The listing builds one solid part. Answer for the finished solid, in the listing's coordinates (mm). Face numbers are marked on the shaded views. Round coordinates to 2 decimals unless told otherwise and drop trailing zeros. Write each loop counter-clockwise with the first axis right and the second up, starting at its lowest first coordinate (ties: lowest second). Pieces come first, ordered by that corner, then holes.
from build123d import *

# Parameters (mm, degrees)
SKETCH1_R                = 36
BOSS_EXTRUDE1_DEPTH      = 5
SKETCH2_R                = 15
CUT_EXTRUDE1_DEPTH       = 5
CUT_EXTRUDE3_DEPTH       = 5
FILLET1_R                = 1.5
CIRPATTERN1_COUNT        = 6
FILLET1_OF_CIRPATTERN1_R = 1.5
SKETCH4_R                = 1.55
CUT_EXTRUDE4_DEPTH       = 5
CIRPATTERN2_COUNT        = 8
BOSS_EXTRUDE2_DEPTH      = 2
CIRPATTERN3_COUNT        = 4


with BuildPart() as part:
    # Sketch1 → Boss-Extrude1 (new body)
    with BuildSketch(Plane(origin=(0, 0, 0), x_dir=(1, 0, 0), z_dir=(0, 1, 0))):
        with Locations(Location((0, 0, 0), (0, 0, 270))):
            Circle(SKETCH1_R)
    extrude(amount=BOSS_EXTRUDE1_DEPTH)

    # Sketch2 → Cut-Extrude1 (cut)
    with BuildSketch(Plane(origin=(0, 5, 0), x_dir=(1, 0, 0), z_dir=(0, 1, 0))):
        with Locations(Location((0, 0, 0), (0, 0, 270))):
            Circle(SKETCH2_R)
    extrude(amount=-CUT_EXTRUDE1_DEPTH, mode=Mode.SUBTRACT)

    # Sketch3 → Cut-Extrude3 (cut)
    with BuildSketch(Plane(origin=(0, 5, 0), x_dir=(1, 0, 0), z_dir=(0, 1, 0))):
        with BuildLine():
            Line((-15.909902577, 15.909902577), (-19.445436483, 19.445436483))
            ThreePointArc((-19.445436483, 19.445436483), (-13.75, 23.815698604), (-7.11752374, 26.562960223))
            Line((-7.11752374, 26.562960223), (-5.823428515, 21.733331092))
            ThreePointArc((-5.823428515, 21.733331092), (-11.25, 19.485571585), (-15.909902577, 15.909902577))
        make_face()
    cut_extrude3 = extrude(amount=-CUT_EXTRUDE3_DEPTH, mode=Mode.SUBTRACT)

    # Fillet1
    fillet1_edges = [part.edges().sort_by_distance(p)[0] for p in [
        (-19.445436483, 2.5, -19.445436483),
        (-7.11752374, 2.5, -26.562960223),
        (-5.823428515, 2.5, -21.733331092),
        (-15.909902577, 2.5, -15.909902577),
    ]]
    fillet(fillet1_edges, radius=FILLET1_R)

    # CirPattern1: Cut-Extrude3 ×6 about axis
    cirpattern1_axis = Axis((0, 0, 0), (0, 1, 0))
    for i in range(1, CIRPATTERN1_COUNT):
        add(cut_extrude3.rotate(cirpattern1_axis, i * 360 / CIRPATTERN1_COUNT), mode=Mode.SUBTRACT)

    # Fillet1 of CirPattern1
    fillet1_of_cirpattern1_edges = [part.edges().sort_by_distance(p)[0] for p in [
        (-26.562960223, 2.5, 7.11752374),
        (-26.562960223, 2.5, -7.11752374),
        (-21.733331092, 2.5, -5.823428515),
        (-21.733331092, 2.5, 5.823428515),
        (-7.11752374, 2.5, 26.562960223),
        (-19.445436483, 2.5, 19.445436483),
        (-15.909902577, 2.5, 15.909902577),
        (-5.823428515, 2.5, 21.733331092),
        (19.445436483, 2.5, 19.445436483),
        (7.11752374, 2.5, 26.562960223),
        (5.823428515, 2.5, 21.733331092),
        (15.909902577, 2.5, 15.909902577),
        (26.562960223, 2.5, -7.11752374),
        (26.562960223, 2.5, 7.11752374),
        (21.733331092, 2.5, 5.823428515),
        (21.733331092, 2.5, -5.823428515),
        (7.11752374, 2.5, -26.562960223),
        (19.445436483, 2.5, -19.445436483),
        (15.909902577, 2.5, -15.909902577),
        (5.823428515, 2.5, -21.733331092),
    ]]
    fillet(fillet1_of_cirpattern1_edges, radius=FILLET1_OF_CIRPATTERN1_R)

    # Sketch4 → Cut-Extrude4 (cut)
    with BuildSketch(Plane(origin=(0, 5, 0), x_dir=(1, 0, 0), z_dir=(0, 1, 0))):
        with Locations(Location((0, 33, 0), (0, 0, 270))):
            Circle(SKETCH4_R)
    cut_extrude4 = extrude(amount=-CUT_EXTRUDE4_DEPTH, mode=Mode.SUBTRACT)

    # CirPattern2: Cut-Extrude4 ×8 about axis
    cirpattern2_axis = Axis((0, 0, 0), (0, 1, 0))
    for i in range(1, CIRPATTERN2_COUNT):
        add(cut_extrude4.rotate(cirpattern2_axis, i * 360 / CIRPATTERN2_COUNT), mode=Mode.SUBTRACT)

    # Sketch6 → Boss-Extrude2 (add)
    with BuildSketch(Plane(origin=(0, 5, 0), x_dir=(1, 0, 0), z_dir=(0, 1, 0))):
        with BuildLine():
            Line((-16.387638055, 25.723439097), (-17.40850731, 27.325882844))
            ThreePointArc((-17.40850731, 27.325882844), (-12.398943209, 29.933696853), (-7.012643492, 31.631990631))
            Line((-7.012643492, 31.631990631), (-6.601408225, 29.777028217))
            ThreePointArc((-6.601408225, 29.777028217), (-11.671844687, 28.178325742), (-16.387638055, 25.723439097))
        make_face()
    boss_extrude2 = extrude(amount=BOSS_EXTRUDE2_DEPTH)

    # CirPattern3: Boss-Extrude2 ×4 about axis
    cirpattern3_axis = Axis((0, 5, 0), (0, -1, 0))
    for i in range(1, CIRPATTERN3_COUNT):
        add(boss_extrude2.rotate(cirpattern3_axis, i * 360 / CIRPATTERN3_COUNT))


solid = part.part
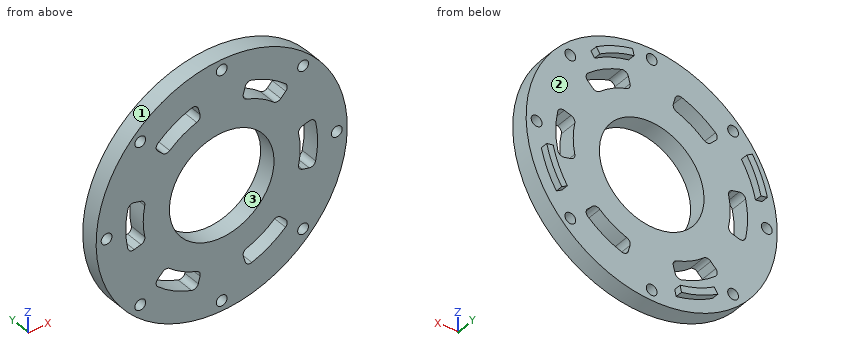
1. For a pull along Z with two mould halves and no side action, classify the marked faces 1, 2 and 3 as released by +Z, released by -Z, zero draft, split by the parting line, or undercut.
Geometry says:
face 1: split by the parting line
face 2: zero draft
face 3: undercut
2. Given pin 1 (1.5 mm diameter, centred on y = 6, z = 13.5, fed in from +X); pin 2 (4 mm diameter, centred on x = 23.33, z = 23.33, fed in from +Y); pin 3 (4 mm diameter, centred on y = 1.5, z = 27, fed in from -X), each flat-ended and moving along its own axis, determine where each tip first touches the part or whether it passes through.
Geometry says:
pin 1: stops at x = -26.97
pin 2: stops at y = 5
pin 3: stops at x = -25.9
3. Section A-A on z = 0 is taken. Determine the outline of the cut face in (x, y).
Geometry says:
outline: (-36, 0) - (-34.55, 0) - (-34.55, 5) - (-36, 5) - close; (-31.45, 0) - (-27.5, 0) - (-27.5, 5) - (-31.45, 5) - close; (-22.5, 0) - (-15, 0) - (-15, 5) - (-22.5, 5) - close; (15, 0) - (22.5, 0) - (22.5, 5) - (15, 5) - close; (27.5, 0) - (31.45, 0) - (31.45, 5) - (27.5, 5) - close; (34.55, 0) - (36, 0) - (36, 5) - (34.55, 5) - close
4. Section B-B on x = 0 is taken. Determine the outline of the cut face in (y, z), plus the area to 3 significant figures.
Geometry says:
outline: (0, -36) - (5, -36) - (5, -34.55) - (0, -34.55) - close; (0, -31.45) - (5, -31.45) - (5, -15) - (0, -15) - close; (0, 15) - (5, 15) - (5, 31.45) - (0, 31.45) - close; (0, 34.55) - (5, 34.55) - (5, 36) - (0, 36) - close
area: 179 mm2
5. Section C-C on z = -33 is taken. Determine the outline of the cut face in (x, y).
Geometry says:
outline: (-14.39, 0) - (-1.55, 0) - (-1.55, 5) - (-14.39, 5) - close; (1.55, 0) - (14.39, 0) - (14.39, 5) - (1.55, 5) - close
6. Straight lines are drawn through the part: line 1 along Z through (x, y) = (-13.5, 3); line 2 along X through (y, z) = (4.25, 18.5); line 3 along X through (y, z) = (4.25, 6). For each, find the intervals that lie inside material, in ascending order.
Geometry says:
line 1: z = -33.37 to -23.96, -18 to -6.54, 6.54 to 18, 23.96 to 33.37
line 2: x = -30.88 to -18.48, -12.81 to 12.81, 18.48 to 30.88
line 3: x = -35.5 to -26.77, -22.7 to -13.75, 13.75 to 22.7, 26.77 to 35.5
7. Section D-D on x = 33 is taken. Determine the outline of the cut face in (y, z).
Geometry says:
outline: (0, -14.39) - (5, -14.39) - (5, -1.55) - (0, -1.55) - close; (0, 1.55) - (5, 1.55) - (5, 14.39) - (0, 14.39) - close
